from build123d import *

# Parameters (mm, degrees)
PAD_DEPTH = 2.5


with BuildPart() as part:
    # Sketch → Pad (new body, symmetric)
    with BuildSketch(Plane.XY):
        Polygon((-140, 137.5), (-70, 137.5), (-70, 45), (70, 45), (70, 137.5), (140, 137.5), (140, -137.5), (70, -137.5), (70, -45), (-70, -45), (-70, -137.5), (-140, -137.5), align=None)
    extrude(amount=PAD_DEPTH, both=True)


solid = part.part
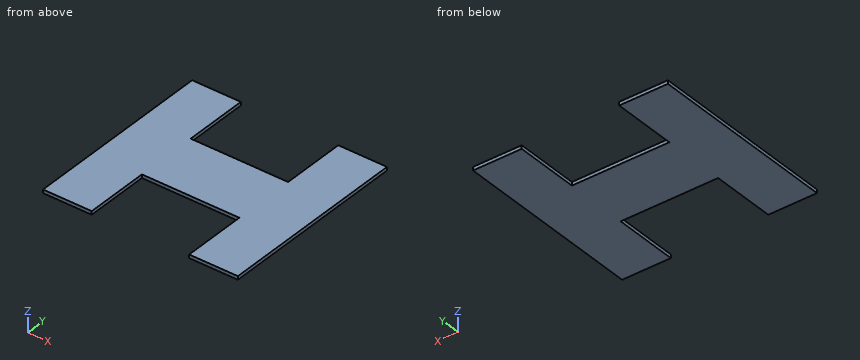
The listing builds one solid part. Answer for the finished solid, in the listing's coordinates (mm). Round coordinates to 2 decimals unless told otherwise and drop trailing zeros. Write each loop counter-clockwise with the first axis right and the second up, starting at its lowest first coordinate (ties: lowest second). Pieces come first, ordered by that corner, then holes. Notation, with made-up numbers: (78, 25.25) - (124, 25.25) arc R19 ccw to (124, 46.25) - close; hole circle Ø6 at (-10, 60.5). An arc over 180 degrees is marked (long way). Use a Markdown table: item, result. Add a question column.
1. A flat-ended cylindrical pin translates along its axis: P1, Ø1.5, axis at x = 29, z = 1, coming from the -Y side. Find the tip coordinate at first contact, or state that the pin passes through.
2. The part is cut by section A-A (y = 64). Write down the section's boundary in (x, z).
3. The part is cut by section B-B (z = 0.35). Write down the section's boundary in (x, y), and give its area (3 significant figures).
4. The part is cut by section C-C (x = -29). Write down the section's boundary in (y, z), and give its area (3 significant figures).
5. Consider line 1 (X direction, y = -70, z = -0.7); line 2 (Y direction, x = -62, z = 0.2). Determine where each line is inside the solid, lowest interval first.
Reported:
| question | item | result |
|---|---|---|
| 1 | P1 | y = -45 |
| 2 | outline | (-140, -2.5) - (-70, -2.5) - (-70, 2.5) - (-140, 2.5) - close; (70, -2.5) - (140, -2.5) - (140, 2.5) - (70, 2.5) - close |
| 3 | outline | (-140, -137.5) - (-70, -137.5) - (-70, -45) - (70, -45) - (70, -137.5) - (140, -137.5) - (140, 137.5) - (70, 137.5) - (70, 45) - (-70, 45) - (-70, 137.5) - (-140, 137.5) - close |
| 3 | area | 51,100 mm^2 |
| 4 | outline | (-45, -2.5) - (45, -2.5) - (45, 2.5) - (-45, 2.5) - close |
| 4 | area | 450 mm^2 |
| 5 | line 1 | -140 to -70, 70 to 140 |
| 5 | line 2 | -45 to 45 |
